Geometry: final body of the model. Coordinates: model frame, mm. Face numbers are marked on the shaded views. A direction names the side the tool comes from. Round coordinates to 2 decimals unless told otherwise and drop trailing zeros. Write each loop counter-clockwise with the first axis right and the second up, starting at its lowest first coordinate (ties: lowest second). Pieces come first, ordered by that corner, then holes. Notation, with made-up numbers: (67, -25.5) -> (96, -25.5) arc R5 cw to (96, -21.5) -> close; hole circle Ø11 at (30.5, -29). An arc over 180 degrees is marked (long way). Use one line per item in the form item = value. Start each with the question number.
1. Cut plane A-A, the plane x = 21.5. Return the cut outline in (y, z).
2. Cut plane C-C, the plane y = 27. Return the cut outline in (x, z).
3. Cut plane D-D, the plane y = 39. Return the cut outline in (x, z).
4. Pin query (flat end, axial travel): pin 1 Ø4 at (x, z) = (6.5, 59) entering from -Y; pin 2 Ø2 at (y, z) = (35, 22.5) entering from +X; pin 3 Ø2.5 at (y, z) = (17, 23.5) entering from +X. Return the tip coordinate at first contact, or that it passes through.
5. Line query: L1, parallel to Z at x = 0, y = 3.5; L2, parallel to Y at x = 7, z = 6; L3, parallel to Y at x = -8, z = 49.5. Output: solid intervals per line, ascending.
6. Draft query along Y for the marked faces 5, 6 and 7. Return one class per face: pulls with the +Y half, pulls with the -Y half, needs draft (parallel to the pull), parting line crosses it, or undercut.
7. Cut plane B-B, the plane y = 18. State how many separate pieces and enclosed holes the cut face has, plus the area to 3 significant figures.
8. Reachability of the marked faces 1, 2, 3 and 4 from +Z, -Z, +X, -X, +Y, -Y: full face, straight path, thin tool, end or side. Return the list, or none.
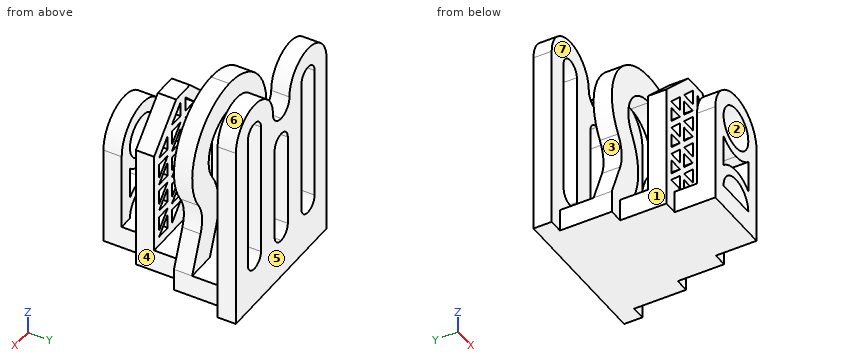
```python
from build123d import *

# Parameters (mm, degrees)
F0_R      = 7.5
F1_DEPTH  = 6.5
F4_DEPTH  = 6.5
F7_DEPTH  = 6.5
F10_DEPTH = 6.5
F12_DEPTH = 8


with BuildPart() as f1:
    # F0 (on Front) → F1 (new body)
    with BuildSketch(Plane.XZ):
        with BuildLine():
            Line((-12.5, 27.5), (-12.5, 0))
            Line((-12.5, 0), (-7.5, 0))
            ThreePointArc((-7.5, 0), (0, 7.5), (7.5, 0))
            Line((7.5, 0), (12.5, 0))
            Line((12.5, 0), (12.5, 27.5))
            ThreePointArc((12.5, 27.5), (0, 40), (-12.5, 27.5))
        make_face()
        with BuildLine():
            Line((-7.5, 13.75), (-7.5, 19.4532615303))
            ThreePointArc((-7.5, 19.4532615303), (-4.0302528973, 17.2649102797), (0, 16.5))
            ThreePointArc((0, 16.5), (4.0302528973, 17.2649102797), (7.5, 19.4532615303))
            Line((7.5, 19.4532615303), (7.5, 13.75))
            Line((7.5, 13.75), (7.5, 8.0467384697))
            ThreePointArc((7.5, 8.0467384697), (4.0302528973, 10.2350897203), (0, 11))
            ThreePointArc((0, 11), (-4.0302528973, 10.2350897203), (-7.5, 8.0467384697))
            Line((-7.5, 8.0467384697), (-7.5, 13.75))
        make_face(mode=Mode.SUBTRACT)
        with Locations((0, 27.5)):
            Circle(F0_R, mode=Mode.SUBTRACT)
    extrude(amount=-F1_DEPTH)



with BuildPart() as f4:
    # F3 (on offset) → F4 (new body)
    with BuildSketch(Plane(origin=(0, 14.5, 0), x_dir=(-1, 0, 0), z_dir=(0, 1, 0))):
        Polygon((-17.5, 0), (17.5, 0), (17.5, 36.6568542495), (4.1568542495, 50), (0, 50), (-4.1568542495, 50), (-17.5, 36.6568542495), align=None)
        Polygon((-14.5, 3.25), (-9.25, 8.5), (-9.25, 3.25), align=None, mode=Mode.SUBTRACT)
        Polygon((-14.5, 11), (-9.25, 11), (-14.5, 5.75), align=None, mode=Mode.SUBTRACT)
        Polygon((-6.75, 3.25), (-6.75, 8.5), (-1.5, 8.5), align=None, mode=Mode.SUBTRACT)
        Polygon((-14.5, 13.5), (-9.25, 18.75), (-9.25, 13.5), align=None, mode=Mode.SUBTRACT)
        Polygon((-14.5, 21.25), (-9.25, 21.25), (-14.5, 16), align=None, mode=Mode.SUBTRACT)
        Polygon((-6.75, 11), (-1.5, 16.25), (-1.5, 11), align=None, mode=Mode.SUBTRACT)
        Polygon((-6.75, 13.5), (-6.75, 18.75), (-1.5, 18.75), align=None, mode=Mode.SUBTRACT)
        Polygon((-6.75, 21.25), (-1.5, 26.5), (-1.5, 21.25), align=None, mode=Mode.SUBTRACT)
        Polygon((6.75, 8.5), (6.75, 3.25), (1.5, 8.5), align=None, mode=Mode.SUBTRACT)
        Polygon((9.25, 8.5), (14.5, 3.25), (9.25, 3.25), align=None, mode=Mode.SUBTRACT)
        Polygon((14.5, 5.75), (9.25, 11), (14.5, 11), align=None, mode=Mode.SUBTRACT)
        Polygon((1.5, 11), (1.5, 16.25), (6.75, 11), align=None, mode=Mode.SUBTRACT)
        Polygon((1.5, 18.75), (6.75, 18.75), (6.75, 13.5), align=None, mode=Mode.SUBTRACT)
        Polygon((1.5, 21.25), (1.5, 26.5), (6.75, 21.25), align=None, mode=Mode.SUBTRACT)
        Polygon((9.25, 13.5), (9.25, 18.75), (14.5, 13.5), align=None, mode=Mode.SUBTRACT)
        Polygon((14.5, 16), (9.25, 21.25), (14.5, 21.25), align=None, mode=Mode.SUBTRACT)
        Polygon((-14.5, 23.75), (-9.25, 29), (-9.25, 23.75), align=None, mode=Mode.SUBTRACT)
        Polygon((-14.5, 31.5), (-9.25, 31.5), (-14.5, 26.25), align=None, mode=Mode.SUBTRACT)
        Polygon((-14.5, 34), (-9.25, 39.25), (-9.25, 34), align=None, mode=Mode.SUBTRACT)
        Polygon((-6.75, 23.75), (-6.75, 29), (-1.5, 29), align=None, mode=Mode.SUBTRACT)
        Polygon((-6.75, 31.5), (-1.5, 36.75), (-1.5, 31.5), align=None, mode=Mode.SUBTRACT)
        Polygon((-6.75, 34), (-6.75, 39.25), (-1.5, 39.25), align=None, mode=Mode.SUBTRACT)
        Polygon((-1.5, 41.75), (-6.75, 41.75), (-1.5, 47), align=None, mode=Mode.SUBTRACT)
        Polygon((1.5, 29), (6.75, 29), (6.75, 23.75), align=None, mode=Mode.SUBTRACT)
        Polygon((1.5, 31.5), (1.5, 36.75), (6.75, 31.5), align=None, mode=Mode.SUBTRACT)
        Polygon((1.5, 39.25), (6.75, 39.25), (6.75, 34), align=None, mode=Mode.SUBTRACT)
        Polygon((9.25, 23.75), (9.25, 29), (14.5, 23.75), align=None, mode=Mode.SUBTRACT)
        Polygon((14.5, 26.25), (9.25, 31.5), (14.5, 31.5), align=None, mode=Mode.SUBTRACT)
        Polygon((9.25, 34), (9.25, 39.25), (14.5, 34), align=None, mode=Mode.SUBTRACT)
        Polygon((1.5, 41.75), (1.5, 47), (6.75, 41.75), align=None, mode=Mode.SUBTRACT)
    extrude(amount=F4_DEPTH)


with BuildPart() as f7:
    # F6 (on offset) → F7 (new body)
    with BuildSketch(Plane(origin=(0, 31, 0), x_dir=(-1, 0, 0), z_dir=(0, 1, 0))):
        with BuildLine():
            ThreePointArc((18.6993614774, 24.9866519133), (19.8469182992, 48.099520462), (0, 60))
            ThreePointArc((0, 60), (-19.8469182992, 48.099520462), (-18.6993614774, 24.9866519133))
            ThreePointArc((-18.6993614774, 24.9866519133), (-16.5755735728, 19.1462143394), (-17.4007867797, 12.9866519133))
            Line((-17.4007867797, 12.9866519133), (-22.5, 0))
            Line((-22.5, 0), (-11.756749629, 0))
            Line((-11.756749629, 0), (-8.0926168547, 9.3317958769))
            ThreePointArc((-8.0926168547, 9.3317958769), (-6.6336162435, 20.2220788589), (-10.3885341541, 30.5481399518))
            ThreePointArc((-10.3885341541, 30.5481399518), (-11.0260657218, 43.3886224789), (0, 50))
            ThreePointArc((0, 50), (11.0260657218, 43.3886224789), (10.3885341541, 30.5481399518))
            ThreePointArc((10.3885341541, 30.5481399518), (6.6336162435, 20.2220788589), (8.0926168547, 9.3317958769))
            Line((8.0926168547, 9.3317958769), (11.756749629, 0))
            Line((11.756749629, 0), (22.5, 0))
            Line((22.5, 0), (17.4007867797, 12.9866519133))
            ThreePointArc((17.4007867797, 12.9866519133), (16.5755735728, 19.1462143394), (18.6993614774, 24.9866519133))
        make_face()
    extrude(amount=F7_DEPTH)


with BuildPart() as f10:
    # F9 (on offset) → F10 (new body)
    with BuildSketch(Plane(origin=(0, 49.5, 0), x_dir=(-1, 0, 0), z_dir=(0, 1, 0))):
        with BuildLine():
            Line((-27.5, 0), (27.5, 0))
            Line((27.5, 0), (27.5, 58.75))
            ThreePointArc((27.5, 58.75), (16.25, 70), (5, 58.75))
            ThreePointArc((5, 58.75), (3.5355339059, 55.2144660941), (0, 53.75))
            ThreePointArc((0, 53.75), (-3.5355339059, 55.2144660941), (-5, 58.75))
            ThreePointArc((-5, 58.75), (-16.25, 70), (-27.5, 58.75))
            Line((-27.5, 58.75), (-27.5, 0))
        make_face()
        with BuildLine():
            ThreePointArc((-20.25, 58.75), (-16.25, 62.75), (-12.25, 58.75))
            Line((-12.25, 58.75), (-12.25, 10))
            ThreePointArc((-12.25, 10), (-16.25, 6), (-20.25, 10))
            Line((-20.25, 10), (-20.25, 58.75))
        make_face(mode=Mode.SUBTRACT)
        with BuildLine():
            ThreePointArc((-4, 43.75), (-2.8284271247, 46.5784271247), (0, 47.75))
            ThreePointArc((0, 47.75), (2.8284271247, 46.5784271247), (4, 43.75))
            Line((4, 43.75), (4, 10))
            ThreePointArc((4, 10), (2.8284271247, 7.1715728753), (0, 6))
            ThreePointArc((0, 6), (-2.8284271247, 7.1715728753), (-4, 10))
            Line((-4, 10), (-4, 43.75))
        make_face(mode=Mode.SUBTRACT)
        with BuildLine():
            ThreePointArc((12.25, 58.75), (16.25, 62.75), (20.25, 58.75))
            Line((20.25, 58.75), (20.25, 10))
            ThreePointArc((20.25, 10), (16.25, 6), (12.25, 10))
            Line((12.25, 10), (12.25, 58.75))
        make_face(mode=Mode.SUBTRACT)
    extrude(amount=F10_DEPTH)


with BuildPart() as f1_1:
    add(f1.part)

    add(f4.part)  # F12 merges F4

    add(f7.part)  # F12 merges F7

    add(f10.part)  # F12 merges F10
    # F11 (on Top) → F12 (join)
    with BuildSketch(Plane.XY):
        Polygon((-12.5, 0), (0, 0), (12.5, 0), (12.5, 6.5), (12.5, 14.5), (17.5, 14.5), (17.5, 21), (17.5, 31), (22.5, 31), (22.5, 37.5), (22.5, 49.5), (27.5, 49.5), (27.5, 56), (0, 56), (-27.5, 56), (-27.5, 49.5), (-22.5, 49.5), (-22.5, 37.5), (-22.5, 31), (-17.5, 31), (-17.5, 21), (-17.5, 14.5), (-12.5, 14.5), (-12.5, 6.5), align=None)
    extrude(amount=-F12_DEPTH)


solid = f1_1.part
```
Outcome:
q1.outline = (31, -8) -> (56, -8) -> (56, 68.7) -> (49.5, 68.7) -> (49.5, 0) -> (37.5, 0) -> (37.5, 2.55) -> (31, 2.55) -> close; (31, 30.87) -> (37.5, 30.87) -> (37.5, 44.13) -> (31, 44.13) -> close
q2.outline = (-17.5, -8) -> (17.5, -8) -> (17.5, 0) -> (-17.5, 0) -> close
q3.outline = (-22.5, -8) -> (22.5, -8) -> (22.5, 0) -> (-22.5, 0) -> close
q4.pin_1 = 31
q4.pin_2 = 17.84
q4.pin_3 = 17.5
q5.L1 = -8 to 0, 7.5 to 11, 16.5 to 20, 35 to 40
q5.L2 = 0 to 6.5, 14.5 to 21, 49.5 to 56
q5.L3 = 31 to 37.5, 49.5 to 56
q6.face_5 = pulls with the +Y half
q6.face_6 = needs draft
q6.face_7 = undercut
q7.separate_pieces = 1
q7.enclosed_holes = 30
q7.area = 1,440 mm^2
q8.face_1 = +Z, -Z, -X, -Y
q8.face_2 = -Y
q8.face_3 = -X, +Y
q8.face_4 = +Z, -Z, +X, -Y
